Check sheet for the modelled part. Datum: model origin and axes. Units: mm. Face numbers are marked on the shaded views. A direction names the side the tool comes from. Round coordinates to 2 decimals unless told otherwise and drop trailing zeros. Order: outer loops, then holes, each group sorted by start corner. A loop starts at its lowest first (then second) coordinate and runs counter-clockwise, first axis right, second up.
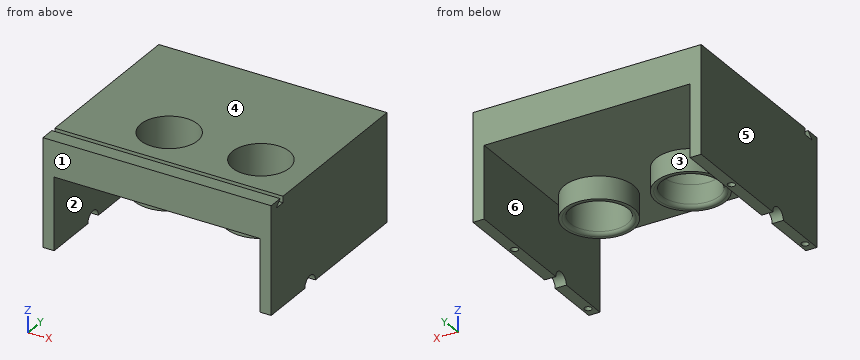
```python
from build123d import *

# Parameters (mm, degrees)
SKETCH2_W           = 102
SKETCH2_H           = 96.13
SKETCH2_W_2         = 92
SKETCH2_H_2         = 64.53
BOSS_EXTRUDE1_DEPTH = 85
SKETCH8_R           = 12.7
CUT_EXTRUDE7_DEPTH  = 20
SKETCH9_R           = 10
CUT_EXTRUDE8_DEPTH  = 20
SKETCH10_R          = 3.875
CUT_EXTRUDE9_DEPTH  = 142.206388754
SKETCH11_W          = 48.065
SKETCH11_H          = 85
CUT_EXTRUDE11_DEPTH = 142.206388754
SKETCH12_R          = 1.6
CUT_EXTRUDE12_DEPTH = 10
SKETCH14_R          = 15.5
SKETCH14_R_2        = 12.7
BOSS_EXTRUDE2_DEPTH = 10
FILLET1_R           = 1.5
CUT_EXTRUDE13_DEPTH = 142.206388754


with BuildPart() as part:
    # Sketch2 → Boss-Extrude1 (new body)
    with BuildSketch(Plane(origin=(0, 0, 0), x_dir=(1, 0, 0), z_dir=(0, 1, 0))):
        Rectangle(SKETCH2_W, SKETCH2_H)
        Rectangle(SKETCH2_W_2, SKETCH2_H_2, mode=Mode.SUBTRACT)
    extrude(amount=BOSS_EXTRUDE1_DEPTH)

    # Sketch8 → Cut-Extrude7 (cut)
    with BuildSketch(Plane.XY.offset(48.065)):
        with Locations((-12, 28.575)):
            Circle(SKETCH8_R)
        with Locations((29, 28.575)):
            Circle(SKETCH8_R)
    extrude(amount=-CUT_EXTRUDE7_DEPTH, mode=Mode.SUBTRACT)

    # Sketch9 → Cut-Extrude8 (cut)
    with BuildSketch(Plane(origin=(0, 0, -48.065), x_dir=(-1, 0, 0), z_dir=(0, 0, -1))):
        with Locations((-31, 31.7)):
            Circle(SKETCH9_R)
        with Locations((29, 31.7)):
            Circle(SKETCH9_R)
    extrude(amount=-CUT_EXTRUDE8_DEPTH, mode=Mode.SUBTRACT)

    # Sketch10 → Cut-Extrude9 (cut, through all)
    with BuildSketch(Plane.ZY.offset(51)):
        with Locations((0, 28.575)):
            Circle(SKETCH10_R)
    extrude(amount=-CUT_EXTRUDE9_DEPTH, mode=Mode.SUBTRACT)

    # Sketch11 → Cut-Extrude11 (cut, through all)
    with BuildSketch(Plane.ZY.offset(51)):
        with Locations((-24.0325, 42.5)):
            Rectangle(SKETCH11_W, SKETCH11_H)
    extrude(amount=-CUT_EXTRUDE11_DEPTH, mode=Mode.SUBTRACT)

    # Sketch12 → Cut-Extrude12 (cut)
    with BuildSketch(Plane(origin=(0, 0, 0), x_dir=(-1, 0, 0), z_dir=(0, 0, -1))):
        with Locations(Location((-48.5, 58.725, 0), (0, 0, 90))):
            Circle(SKETCH12_R)
        with Locations(Location((-48.5, 4.675, 0), (0, 0, 270))):
            Circle(SKETCH12_R)
        with Locations(Location((48.5, 4.675, 0), (0, 0, 90))):
            Circle(SKETCH12_R)
        with Locations(Location((48.5, 58.725, 0), (0, 0, 270))):
            Circle(SKETCH12_R)
    extrude(amount=-CUT_EXTRUDE12_DEPTH, mode=Mode.SUBTRACT)

    # Sketch14 → Boss-Extrude2 (add)
    # profile 1 of 2: a face of its own
    with BuildSketch(Plane(origin=(0, 0, 32.265), x_dir=(-1, 0, 0), z_dir=(0, 0, -1))):
        with Locations((-29, 28.575)):
            Circle(SKETCH14_R)
        with Locations(Location((-29, 28.575, 0), (0, 0, 180))):
            Circle(SKETCH14_R_2, mode=Mode.SUBTRACT)
    # profile 2 of 2: a face of its own
    with BuildSketch(Plane(origin=(0, 0, 32.265), x_dir=(-1, 0, 0), z_dir=(0, 0, -1))):
        with Locations((12, 28.575)):
            Circle(SKETCH14_R)
        with Locations(Location((12, 28.575, 0), (0, 0, 180))):
            Circle(SKETCH14_R_2, mode=Mode.SUBTRACT)
    extrude(amount=BOSS_EXTRUDE2_DEPTH)

    # Fillet1
    fillet1_edges = [part.edges().sort_by_distance(p)[0] for p in [
        (16.3, 28.575, 22.265),
        (-24.7, 28.575, 22.265),
    ]]
    fillet(fillet1_edges, radius=FILLET1_R)

    # Sketch15 → Cut-Extrude13 (cut, through all)
    with BuildSketch(Plane(origin=(51, 0, 0), x_dir=(0, 0, -1), z_dir=(1, 0, 0))):
        Polygon((-48.065, 6.5), (-45.236572875, 3.671572875), (-45.236572875, 8.671572875), (-48.065, 8.671572875), align=None)
    extrude(amount=-CUT_EXTRUDE13_DEPTH, mode=Mode.SUBTRACT)


solid = part.part
```
Item 1: Sectioned sample at A-A (x = -12). Record the cut outline in (y, z) (3 decimals).
Answer:
outline: (0, 32.265) - (13.075, 32.265) - (13.075, 22.265) - (14.375, 22.265) arc R1.5 ccw to (15.875, 23.765) - (15.875, 48.065) - (8.672, 48.065) - (8.672, 45.237) - (3.672, 45.237) - (6.5, 48.065) - (0, 48.065) - close; (41.275, 23.765) arc R1.5 ccw to (42.775, 22.265) - (44.075, 22.265) - (44.075, 32.265) - (85, 32.265) - (85, 48.065) - (41.275, 48.065) - close
Item 2: Release check for a two-part mould opening along X. For the marked faces 4, 5 and 6 record: released by +X, released by -X, zero draft, split by the parting line, or undercut.
Answer:
face 4: zero draft
face 5: released by -X
face 6: undercut
Item 3: Access from +Z, -Z, +X, -X, +Y, -Y to the whole of each face (thin tool, end or side, straight path). Record for the marked faces 1, 2 and 3.
Answer:
face 1: +Z, -Z, +X, -X, -Y
face 2: -Z, +Y, -Y
face 3: -Z
Item 4: Sectioned sample at C-C (z = 26.5). Record the cut outline in (x, y) (3 decimals), and give its area (3 significant figures).
Answer:
outline: (-51, 0) - (-46, 0) - (-46, 85) - (-51, 85) - close; circle Ø31 at (-12, 28.575); circle Ø31 at (29, 28.575); (46, 0) - (51, 0) - (51, 85) - (46, 85) - close; hole circle Ø25.4 at (-12, 28.575); hole circle Ø25.4 at (29, 28.575)
area: 1,350 mm2
Item 5: Scan lines: line 1 along Y through (x, z) = (29.5, 30); line 2 along X through (y, z) = (21.5, 16.5); line 3 along Y through (x, z) = (29, 42) (3 decimals). Record each from-to range of solid material in increasing order.
Answer:
line 1: y = 13.08 to 15.88, 41.27 to 44.07
line 2: x = -51 to -46, 46 to 51
line 3: y = 0 to 15.875, 41.275 to 85
Item 6: Go/stop test with flat-tipped pins: P1, Ø3, axis at x = -22, y = 43.5, coming from the -Z side (3 decimals); P2, Ø25, axis at x = -14, y = 34, coming from the -Z side (3 decimals); P3, Ø1, axis at x = 48, y = 5, coming from the -Z side. Record where each tip stops, or that it passes through.
Answer:
P1: stops at z = 32.265
P2: stops at z = 22.265
P3: stops at z = 10
Item 7: Sectioned sample at D-D (x = 12). Record the cut outline in (y, z) (3 decimals), and give its area (3 significant figures).
Answer:
outline: (0, 32.265) - (85, 32.265) - (85, 48.065) - (8.672, 48.065) - (8.672, 45.237) - (3.672, 45.237) - (6.5, 48.065) - (0, 48.065) - close
area: 1,330 mm2
Item 8: Sectioned sample at B-B (z = 16.5). Record the cut outline in (x, y).
Answer:
outline: (-51, 0) - (-46, 0) - (-46, 85) - (-51, 85) - close; (46, 0) - (51, 0) - (51, 85) - (46, 85) - close
